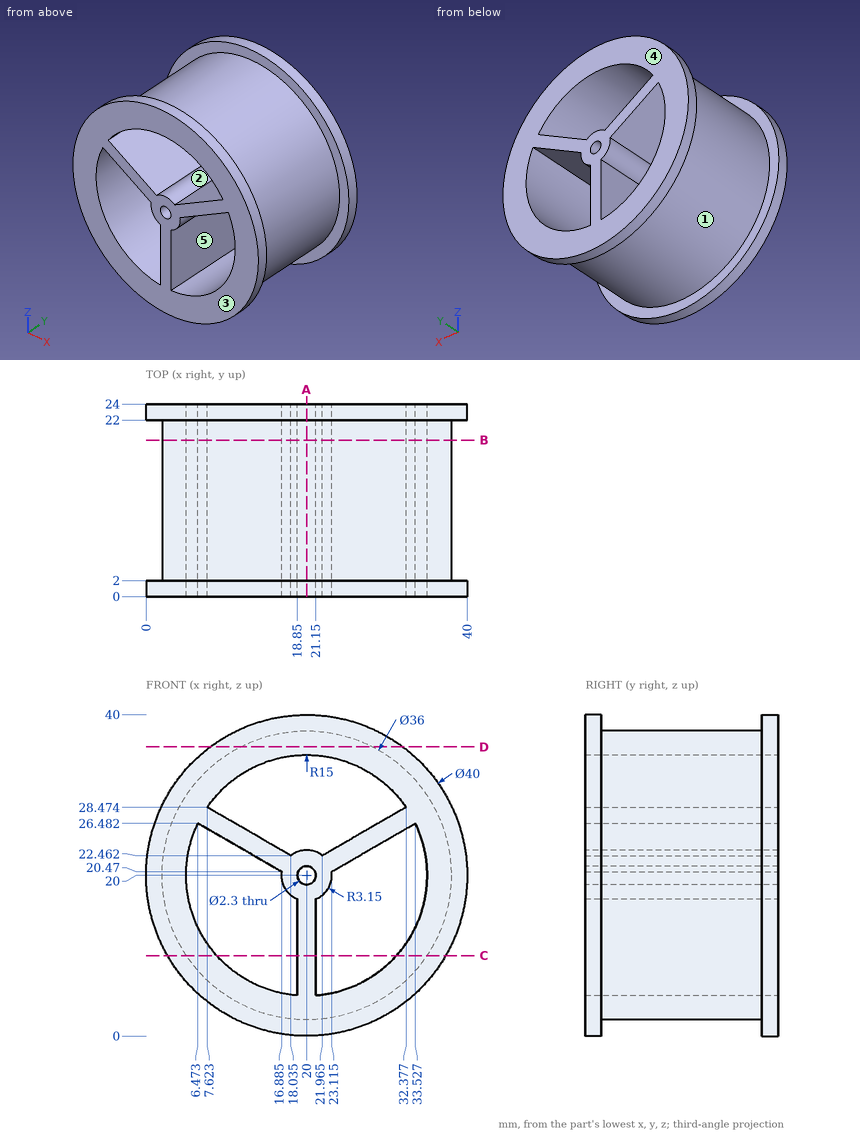
Geometry check sheet. Reference: drawing and pictorial views, mm from the part's lowest x, y, z. A direction names the side the tool comes from. Give positions to 0.01 mm unless a question says otherwise; leave off trailing zeros. Order: outer loops, then holes, each group sorted by start corner. A loop starts at its lowest first (then second) coordinate and runs counter-clockwise, first axis right, second up. Notation, with made-up numbers: M 3,-21.75 L 43,-21.75 A14 cw 43,-2.75 Z; hole C 6,-6.5 d4. An arc over 180 degrees is marked long. Return JSON: item names as keys, results as strings. Group by question number.
1) Section check D-D on z = 36. Record the cut outline in (x, y), and give its area (3 significant figures).
2) Section check B-B on y = 19.5. Give the number of separate pieces and of enclosed holes in the cut face, and give its area (3 significant figures).
3) Section check C-C on z = 10. Record the cut outline in (x, y).
4) Scan lines: line 1 (Z direction, x = 20, y = 14.5); line 2 (X direction, y = 8.25, z = 20); line 3 (Y direction, x = 33.5, z = 8). Record each from-to range of solid material in increasing order.
5) Access from +Z, -Z, +X, -X, +Y, -Y to the whole of each face (thin tool, end or side, straight path). Record for the marked faces 4 and 5.
6) Section check A-A on x = 20. Record the cut outline in (y, z).
7) Go/stop test with flat-tipped pins: pin 1 Ø1.5 at (x, z) = (27.5, 28.5) entering from +Y; pin 2 Ø1.5 at (x, y) = (23.5, 5) entering from -Z; pin 3 Ø9.5 at (y, z) = (14, 11) entering from +X; pin 4 Ø1.5 at (x, y) = (15.5, 11) entering from -Z (1 decimal). Record where each tip stops, or that it passes through.
8) Mould release check, pull along X, two halves, no side actions. Record for the marked faces 1, 2 and 3: pulls with the +X half, pulls with the -X half, needs draft (parallel to the pull), parting line crosses it, or undercut.
Answer block:
{
 "1": {"outline": "M 8,0 L 32,0 L 32,2 L 28.25,2 L 28.25,22 L 32,22 L 32,24 L 8,24 L 8,22 L 11.75,22 L 11.75,2 L 8,2 Z", "area": "426 mm^2"},
 "2": {"separate pieces": "1", "enclosed holes": "4", "area": "420 mm^2"},
 "3": {"outline": "M 2.68,0 L 8.82,0 L 8.82,24 L 2.68,24 L 2.68,22 L 5.03,22 L 5.03,2 L 2.68,2 Z; M 18.85,0 L 21.15,0 L 21.15,24 L 18.85,24 Z; M 31.18,0 L 37.32,0 L 37.32,2 L 34.97,2 L 34.97,22 L 37.32,22 L 37.32,24 L 31.18,24 Z"},
 "4": {"line 1": "z = 2 to 18.85, 21.15 to 23.15, 35 to 38", "line 2": "x = 2 to 5, 16.85 to 18.85, 21.15 to 23.15, 35 to 38", "line 3": "y = 0 to 2, 22 to 24"},
 "5": {"face 4": "+Z, -Z, +X, -X, +Y", "face 5": "+Y, -Y"},
 "6": {"outline": "M 0,0 L 2,0 L 2,2 L 22,2 L 22,0 L 24,0 L 24,18.85 L 0,18.85 Z; M 0,21.15 L 24,21.15 L 24,23.15 L 0,23.15 Z; M 0,35 L 24,35 L 24,40 L 22,40 L 22,38 L 2,38 L 2,40 L 0,40 Z"},
 "7": {"pin 1": "passes through", "pin 2": "stops at z = 2.21", "pin 3": "stops at x = 37.49", "pin 4": "stops at z = 2.4"},
 "8": {"face 1": "parting line crosses it", "face 2": "undercut", "face 3": "needs draft"}
}
